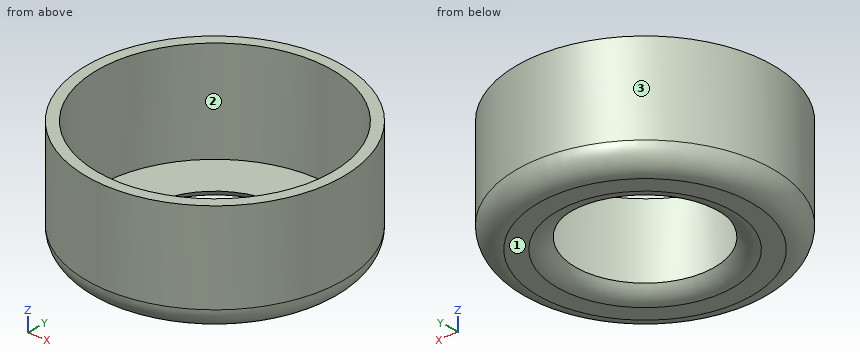
```python
from build123d import *

# Parameters (mm, degrees)
F0_R     = 12
F0_R_2   = 11
F1_DEPTH = 10.5
F2_DEPTH = 1
F3_R     = 6.5
F4_DEPTH = 25


# Not quite as in the source:
# - a fillet or chamfer that OpenCascade refuses, or shapes differently, is made with other operations: its cross-section is extruded or revolved along the edge and cut away or added


with BuildPart() as f1:
    # F0 (on Top) → F1 (new body)
    with BuildSketch(Plane.XY):
        Circle(F0_R)
        Circle(F0_R_2, mode=Mode.SUBTRACT)
    extrude(amount=F1_DEPTH)

    # F0 (on Top) → F2 (join)
    with BuildSketch(Plane.XY):
        Circle(F0_R_2)
    extrude(amount=F2_DEPTH)

    # F3 (on face) → F4 (cut)
    with BuildSketch(Plane.XY):
        Circle(F3_R)
    extrude(amount=F4_DEPTH, mode=Mode.SUBTRACT)

    # F5: fillet of radius 2 on 2 edges, made by hand

    # F5_s1 → F5_t2 (revolve, cut)
    with BuildSketch(Plane.XZ):
        with BuildLine():
            ThreePointArc((12, 2), (11.4142135624, 0.5857864376), (10, 0))
            Line((10, 0), (12, 0))
            Line((12, 0), (12, 2))
        make_face()
    revolve(axis=Axis((0, 0, 0), (0, 0, 1)), mode=Mode.SUBTRACT)

    # F5_s3 → F5_t4 (revolve, cut)
    with BuildSketch(Plane.XZ):
        with BuildLine():
            ThreePointArc((8.2320508076, 0), (7.2320508076, 0.2679491924), (6.5, 1))
            Line((6.5, 1), (6.5, 0))
            Line((6.5, 0), (8.2320508076, 0))
        make_face()
    revolve(axis=Axis((0, 0, 0), (0, 0, 1)), mode=Mode.SUBTRACT)


solid = f1.part
```
Verification items for the finished model (mm, model axes). Face numbers are marked on the shaded views. Coordinates: 2 decimals unless noted, no trailing zeros. Loops run counter-clockwise (first coordinate to the right, second up) from the corner with the lowest first, then second, coordinate; pieces in that order, holes last. Notation, with made-up numbers: (7, 68.5) -> (18, 68.5) arc R27 cw to (18, 107.5) -> close; hole circle Ø2 at (3, 41). An arc over 180 degrees is marked (long way). Answer in a Markdown table with one row per item. Add a question column.
1. Material ranges on probe 1 along Y at (x, z) = (0, 7.75); probe 2 along X at (y, z) = (-7.5, 4.25); probe 3 along Y at (x, z) = (-9.25, 1.5), recorded low to high. Write a range as [from, to].
2. Depth check by flat-ended pin: P1, Ø1, axis at y = -3, z = 4.5, coming from the -X side; P2, Ø5, axis at x = -6, z = 7.5, coming from the -Y side; P3, Ø6, axis at y = -9, z = 5, coming from the -X side. Enter the tip coordinate at first touch or a pass-through.
3. Section check C-C, the plane z = 5.5. Enter the section's corners in (x, y), then the cut area to 3 significant figures.
4. Draft check along X on the marked faces 1, 2 and 3. Enter one of: +X half, -X half, draft (parallel to the pull), parting line (faces both ways), or undercut.
5. Section check A-A, the plane y = 0. Enter the section's corners in (x, z), then the cut area to 3 significant figures.
Derived:
| question | item | result |
|---|---|---|
| 1 | probe 1 | y = [-12, -11], [11, 12] |
| 1 | probe 2 | x = [-9.37, -8.05], [8.05, 9.37] |
| 1 | probe 3 | y = [-7.54, -5.95], [5.95, 7.54] |
| 2 | P1 | stops at x = -11.74 |
| 2 | P2 | stops at y = -11.48 |
| 2 | P3 | stops at x = -10.39 |
| 3 | outline | circle Ø24 at (0, 0); hole circle Ø22 at (0, 0) |
| 3 | area | 72.3 mm² |
| 4 | face 1 | draft |
| 4 | face 2 | undercut |
| 4 | face 3 | parting line |
| 5 | outline | (-12, 2) arc R2 ccw to (-10, 0) -> (-8.23, 0) arc R2 ccw to (-6.5, 1) -> (-11, 1) -> (-11, 10.5) -> (-12, 10.5) -> close; (6.5, 1) arc R2 ccw to (8.23, 0) -> (10, 0) arc R2 ccw to (12, 2) -> (12, 10.5) -> (11, 10.5) -> (11, 1) -> close |
| 5 | area | 27.3 mm² |
